Could you check a few things on this model? Use its own coordinates, in mm. Give positions to 0.01 mm unless a question says otherwise; leave off trailing zeros. Write each loop counter-clockwise with the first axis right and the second up, starting at its lowest first coordinate (ties: lowest second). Pieces come first, ordered by that corner, then holes. Notation, with made-up numbers: M 69,-1.5 L 116,-1.5 A30 cw 116,37.5 Z; hole C -17.5,41 d9. An arc over 180 degrees is marked long. One line per item, written item: value.
```python
from build123d import *

# Parameters (mm, degrees)
BOSS_EXTRUDE1_DEPTH                           = 1.5875
CSK_FOR_8_FLAT_HEAD_SOCKET_CAP_SCREW1_A_COUNT = 2
CSK_FOR_8_FLAT_HEAD_SOCKET_CAP_SCREW1_A_PITCH = 307.345506508


with BuildPart() as part:
    # Sketch2 → Boss-Extrude1 (new body)
    with BuildSketch(Plane(origin=(0, 0, 0), x_dir=(1, 0, 0), z_dir=(0, 1, 0))):
        with BuildLine():
            Line((-148.740503176, 39.854897708), (-164.074575668, 43.963650049))
            ThreePointArc((-164.074575668, 43.963650049), (0, 169.8625), (164.074575668, 43.963650049))
            Line((164.074575668, 43.963650049), (148.740503176, 39.854897708))
            ThreePointArc((148.740503176, 39.854897708), (0, 153.9875), (-148.740503176, 39.854897708))
        make_face()
    extrude(amount=BOSS_EXTRUDE1_DEPTH)

    # Sketch4 → CSK for #8 Flat Head Socket Cap Screw1 (revolve, cut)
    with BuildSketch(Plane(origin=(-153.672753254, 1.5875, -51.033229688), x_dir=(0, 0, 1), z_dir=(1, 0, 0))):
        Polygon((0, 0), (0, 1.5875), (2.2479, 1.5875), (2.2479, 2.658961536), (4.5593, 0), align=None)
    csk_for_8_flat_head_socket_cap_screw1 = revolve(axis=Axis((-153.672753254, 7.9375, -51.033229688), (0, -1, 0)), mode=Mode.SUBTRACT)

    # CSK for #8 Flat Head Socket Cap Screw1 a: CSK for #8 Flat Head Socket Cap Screw1 ×2
    with Locations(*[(i * CSK_FOR_8_FLAT_HEAD_SOCKET_CAP_SCREW1_A_PITCH, 0, 0) for i in range(1, CSK_FOR_8_FLAT_HEAD_SOCKET_CAP_SCREW1_A_COUNT)]):
        add(csk_for_8_flat_head_socket_cap_screw1, mode=Mode.SUBTRACT)


solid = part.part
```
1) If we section it at D-D, the plane x = 31.5: Write out the boundary of the cut face in (y, z).
Outcome:
outline: M 0,-166.92 L 1.59,-166.92 L 1.59,-150.73 L 0,-150.73 Z
2) Please list where these lines run through material, in increasing order: L1, parallel to X at y = 1.4, z = -99.5; L2, parallel to X at y = 0.3, z = -127; L3, parallel to Z at x = -26.5, y = 0.75. Write a range as from..to.
Outcome:
L1: x = -137.67..-117.52, 117.52..137.67
L2: x = -112.8..-87.08, 87.08..112.8
L3: z = -167.78..-151.69
3) If we section it at A-A, the plane z = -82: Write out the boundary of the cut face in (x, y).
Outcome:
outline: M -148.76,0 L -130.34,0 L -130.34,1.59 L -148.76,1.59 Z; M 130.34,0 L 148.76,0 L 148.76,1.59 L 130.34,1.59 Z
4) If we section it at B-B, the plane y = 0.25: Write out the boundary of the cut face in (x, z) (1 decimal), then the cut area to 3 significant figures.
Outcome:
outline: M -164.1,-44 A169.9 ccw 164.1,-44 L 148.7,-39.9 A154 cw -148.7,-39.9 Z; hole C -153.7,-51 d6.8; hole C 153.7,-51 d6.8
area: 6,660 mm^2
5) If we section it at C-C, the plane z = -140: Write out the boundary of the cut face in (x, y).
Outcome:
outline: M -96.19,0 L -64.13,0 L -64.13,1.59 L -96.19,1.59 Z; M 64.13,0 L 96.19,0 L 96.19,1.59 L 64.13,1.59 Z
